Autodesk Inventor part; units mm, degrees
ref_plane "YZ Plane" through (0, 0, 0) normal (1, 0, 0) x (0, 1, 0)
ref_plane "XZ Plane" through (0, 0, 0) normal (0, 1, 0) x (-1, 0, 0)
ref_plane "XY Plane" through (0, 0, 0) normal (0, 0, 1) x (1, 0, 0)
sketch "Sketch4" plane through (0, 0, 0) normal (0, 1, 0) x (-1, 0, 0)
  circle A0 centre (0, 0) radius 12.5
  dimension "d19" = 25
extrude "Extrusion2" add sketch "Sketch4" along normal blind 10
sketch "Sketch5" plane through (0, 0, 0) normal (0, -1, 0) x (1, 0, 0)
  circle A0 centre (0, 0) radius 10
  dimension "d22" = 20
extrude "Extrusion3" add sketch "Sketch5" along normal blind 10
sketch "Sketch6" plane through (0, 10, 0) normal (0, 1, 0) x (1, 0, 0)
  point P0 (0, 0)
  point P1 (0, 0)
hole "Hole2" at (0, 10, 0) direction (0, -1, 0) diameter 3.4587 end through all
equation "\"d30\" = Thickness"
equation "\"BendRadius\" = Thickness"
equation "\"BendReliefWidth\" = Thickness"
equation "\"BendReliefDepth\" = 0.5 * Thickness"
equation "\"CornerReliefSize\" = 4 * Thickness"
equation "\"MinimumRemnant\" = 2 * Thickness"
equation "\"TransitionRadius\" = BendRadius"
equation "\"JacobiRadiusSize\" = BendRadius"
equation "\"GapSize\" = Thickness"
properties part number "Output link probe hub"
CAD build for the part. Positions are in the model's coordinates, mm. A direction names the side the tool comes from. Coordinates: 2 decimals unless noted, no trailing zeros. Loops run counter-clockwise (first coordinate to the right, second up) from the corner with the lowest first, then second, coordinate; pieces in that order, holes last. Notation, with made-up numbers: (81.25, 45.5) - (130.25, 45.5) arc R32 ccw to (130.25, 80.5) - close; hole circle Ø9 at (19, 52.25). An arc over 180 degrees is marked (long way). Use CSV: the item, a comma, the result in double quotes. Start each with the question number.
Q1. Cut at B-B, the plane z = 0. List the corners of the cut face in (x, y).
Q2. Cut at A-A, the plane x = 0. List the corners of the cut face in (y, z), then the cut area to 3 significant figures.
Q3. Drop flat-ended pins along their axis: P1, Ø10, axis at y = 4.5, z = 0.5, coming from the -X side; P2, Ø1, axis at y = -2.5, z = -5.5, coming from the -X side; P3, Ø3, axis at y = -5, z = 3.5, coming from the -X side; P4, Ø1.5, axis at y = -7, z = -9.5, coming from the -X side. Give the stop position or say it passes through.
Q4. Cut at C-C, the plane z = -5. List the corners of the cut face in (x, y).
Q5. Two-plate mould, pull along X, no slides. Class faces 1 (the flat face through (2, -10, 0)), 2 (the cylindrical face through (-2.17, -4.93, 9.76)), 3 (the cylindrical face through (-0.52, -0.14, 1.65)): +X half, -X half, draft (parallel to the pull), parting line (faces both ways), or undercut.
Q6. Probe probe 1 along Z at (x, y) = (0, 3); probe 2 along Z at (x, y) = (0, -5.5); probe 3 along X at (y, z) = (3.5, 1.5). List the from-to ranges inside material, lowest first. Write a range as from..to.
Q7. Cut at D-D, the plane x = 4.75. List the corners of the cut face in (y, z).
Q8. 3-axis set-ups, long thin cutter, end or side, ignore diameter. For faces 4 (the flat face through (0, 10, -3)), 5 (the flat face through (0.1, 0, 10.2)): which of +Z, -Z, +X, -X, +Y, -Y reach the whole face in a straight line?
Here are the results:
1,outline,"(-12.5, 0) - (-10, 0) - (-10, -10) - (-1.73, -10) - (-1.73, 10) - (-12.5, 10) - close; (1.73, -10) - (10, -10) - (10, 0) - (12.5, 0) - (12.5, 10) - (1.73, 10) - close"
2,outline,"(-10, -10) - (0, -10) - (0, -12.5) - (10, -12.5) - (10, -1.73) - (-10, -1.73) - close; (-10, 1.73) - (10, 1.73) - (10, 12.5) - (0, 12.5) - (0, 10) - (-10, 10) - close"
2,area,"381 mm2"
3,P1,"x = -12.5"
3,P2,"x = -8.66"
3,P3,"x = -9.8"
3,P4,"x = -4.84"
4,outline,"(-11.46, 0) - (-8.66, 0) - (-8.66, -10) - (8.66, -10) - (8.66, 0) - (11.46, 0) - (11.46, 10) - (-11.46, 10) - close"
5,face 1,"draft"
5,face 2,"parting line"
5,face 3,"undercut"
6,probe 1,"-12.5..-1.73, 1.73..12.5"
6,probe 2,"-10..-1.73, 1.73..10"
6,probe 3,"-12.41..-0.86, 0.86..12.41"
7,outline,"(-10, -8.8) - (0, -8.8) - (0, -11.56) - (10, -11.56) - (10, 11.56) - (0, 11.56) - (0, 8.8) - (-10, 8.8) - close"
8,face 4,"+Z, -Z, +X, -X, +Y"
8,face 5,"-Y"
